```python
from build123d import *

# Parameters (mm, degrees)
SKETCH1_W                      = 80
SKETCH1_H                      = 40
BOSS_EXTRUDE1_DEPTH            = 1000
BOSS_EXTRUDE1_2_DEPTH          = 1000
BOSS_EXTRUDE1_3_DEPTH          = 1000
BOSS_EXTRUDE1_4_DEPTH          = 1000
BOSS_EXTRUDE1_5_DEPTH          = 1000
BOSS_EXTRUDE1_6_DEPTH          = 1000
SKETCH3_W                      = 880
SKETCH3_H                      = 720
SKETCH3_H_2                    = 400
BOSS_EXTRUDE2_DEPTH            = 40
SKETCH4_W                      = 1040
SKETCH4_H                      = 800
SKETCH4_W_2                    = 880
SKETCH4_H_2                    = 720
BOSS_EXTRUDE4_DEPTH            = 40
SKETCH6_W                      = 2000
SKETCH6_H                      = 800
SKETCH6_W_2                    = 880
SKETCH6_H_2                    = 720
BOSS_EXTRUDE5_DEPTH            = 40
SKETCH7_W                      = 80
SKETCH7_H                      = 40
SKETCH8_W                      = 40
SKETCH8_H                      = 40
SKETCH9_W                      = 80
SKETCH9_H                      = 60
BOSS_EXTRUDE6_DEPTH            = 10
F_10_0_10_DIAMETER_HOLE1_D     = 10
F_10_0_10_DIAMETER_HOLE1_DEPTH = 10
MIRROR5_COPY_1_SKETCH_W        = 80
MIRROR5_COPY_1_SKETCH_H        = 60
MIRROR5_COPY_1_DEPTH           = 10
MIRROR5_COPY_2_D               = 10
MIRROR5_COPY_2_DEPTH           = 10


with BuildPart() as part:
    # Sketch1 → Boss-Extrude1 (new body)
    with BuildSketch(Plane(origin=(0, 0, 0), x_dir=(1, 0, 0), z_dir=(0, 1, 0))):
        with Locations((-960, -380)):
            Rectangle(SKETCH1_W, SKETCH1_H)
    extrude(amount=BOSS_EXTRUDE1_DEPTH)



with BuildPart() as body_2:
    # Sketch1 → Boss-Extrude1 2 (new body)
    with BuildSketch(Plane(origin=(0, 0, 0), x_dir=(1, 0, 0), z_dir=(0, 1, 0))):
        with Locations((0, -380)):
            Rectangle(SKETCH1_W, SKETCH1_H)
    extrude(amount=BOSS_EXTRUDE1_2_DEPTH)


with BuildPart() as body_3:
    # Sketch1 → Boss-Extrude1 3 (new body)
    with BuildSketch(Plane(origin=(0, 0, 0), x_dir=(1, 0, 0), z_dir=(0, 1, 0))):
        with Locations((0, 380)):
            Rectangle(SKETCH1_W, SKETCH1_H)
    extrude(amount=BOSS_EXTRUDE1_3_DEPTH)


with BuildPart() as body_4:
    # Sketch1 → Boss-Extrude1 4 (new body)
    with BuildSketch(Plane(origin=(0, 0, 0), x_dir=(1, 0, 0), z_dir=(0, 1, 0))):
        with Locations((-960, 380)):
            Rectangle(SKETCH1_W, SKETCH1_H)
    extrude(amount=BOSS_EXTRUDE1_4_DEPTH)


with BuildPart() as body_5:
    # Sketch1 → Boss-Extrude1 5 (new body)
    with BuildSketch(Plane(origin=(0, 0, 0), x_dir=(1, 0, 0), z_dir=(0, 1, 0))):
        with Locations((960, -380)):
            Rectangle(SKETCH1_W, SKETCH1_H)
    extrude(amount=BOSS_EXTRUDE1_5_DEPTH)


with BuildPart() as body_6:
    # Sketch1 → Boss-Extrude1 6 (new body)
    with BuildSketch(Plane(origin=(0, 0, 0), x_dir=(1, 0, 0), z_dir=(0, 1, 0))):
        with Locations((960, 380)):
            Rectangle(SKETCH1_W, SKETCH1_H)
    extrude(amount=BOSS_EXTRUDE1_6_DEPTH)


with BuildPart() as part_1:
    add(part.part)

    add(body_2.part)  # Boss-Extrude2 merges body 2

    add(body_3.part)  # Boss-Extrude2 merges body 3

    add(body_4.part)  # Boss-Extrude2 merges body 4

    add(body_5.part)  # Boss-Extrude2 merges body 5

    add(body_6.part)  # Boss-Extrude2 merges body 6
    # Sketch3 → Boss-Extrude2 (add)
    with BuildSketch(Plane(origin=(0, 200, 0), x_dir=(-1, 0, 0), z_dir=(0, -1, 0))):
        Polygon((920, -240), (40, -240), (40, -400), (-1000, -400), (-1000, 400), (40, 400), (40, 240), (920, 240), (920, 400), (1000, 400), (1000, -400.075117412), (920, -400.075117412), align=None)
        with Locations((-480, 0)):
            Rectangle(SKETCH3_W, SKETCH3_H, mode=Mode.SUBTRACT)
        with Locations((480, 0)):
            Rectangle(SKETCH3_W, SKETCH3_H_2, mode=Mode.SUBTRACT)
    extrude(amount=BOSS_EXTRUDE2_DEPTH)

    # Sketch4 → Boss-Extrude4 (add)
    with BuildSketch(Plane(origin=(0, 600, 0), x_dir=(-1, 0, 0), z_dir=(0, -1, 0))):
        with Locations((-480, 0)):
            Rectangle(SKETCH4_W, SKETCH4_H)
        with Locations((-480, 0)):
            Rectangle(SKETCH4_W_2, SKETCH4_H_2, mode=Mode.SUBTRACT)
    extrude(amount=BOSS_EXTRUDE4_DEPTH)

    # Sketch6 → Boss-Extrude5 (add)
    with BuildSketch(Plane(origin=(0, 1000, 0), x_dir=(1, 0, 0), z_dir=(0, 1, 0))):
        Rectangle(SKETCH6_W, SKETCH6_H)
        with Locations((-480, 0)):
            Rectangle(SKETCH6_W_2, SKETCH6_H_2, mode=Mode.SUBTRACT)
        with Locations((480, 0)):
            Rectangle(SKETCH6_W_2, SKETCH6_H_2, mode=Mode.SUBTRACT)
    extrude(amount=BOSS_EXTRUDE5_DEPTH)

    # Sweep1: sweep along a curve in space
    with BuildLine() as sweep1_path:
        Line((-960, 200, 360), (-960, 1000, -360))
    # Sketch7 → Sweep1 (sweep)
    with BuildSketch(Plane(origin=(-960, 200, 360), x_dir=(1, 0, 0), z_dir=(0, 0.7432941462471683, -0.6689647316224475))):
        Rectangle(SKETCH7_W, SKETCH7_H)
    sweep(path=sweep1_path.line)

    # Sweep2: sweep along a curve in space
    with BuildLine() as sweep2_path:
        Line((-40, 200, -380), (-920, 1000, -380))
    # Sketch8 → Sweep2 (sweep)
    with BuildSketch(Plane(origin=(-40, 200, -380), x_dir=(0, 0, 1), z_dir=(-0.7399400733959437, 0.6726727939963126, -3.6407320166765e-15))):
        Rectangle(SKETCH8_W, SKETCH8_H)
    sweep(path=sweep2_path.line)

    # Sketch9 → Boss-Extrude6 (add)
    with BuildSketch(Plane.XZ):
        with Locations((960, -330)):
            Rectangle(SKETCH9_W, SKETCH9_H)
    boss_extrude6 = extrude(amount=-BOSS_EXTRUDE6_DEPTH)

    # Ø10.0 (10) Diameter Hole1
    with Locations(Plane(origin=(0, 10, 0), x_dir=(1, 0, 0), z_dir=(0, 1, 0))):
        with Locations((960, 330)):
            f_10_0_10_diameter_hole1 = Hole(F_10_0_10_DIAMETER_HOLE1_D / 2, depth=F_10_0_10_DIAMETER_HOLE1_DEPTH)

    # Mirror4: Boss-Extrude6, Ø10.0 (10) Diameter Hole1 across plane
    add(boss_extrude6.mirror(Plane.XY))
    add(f_10_0_10_diameter_hole1.mirror(Plane.XY), mode=Mode.SUBTRACT)

    # Mirror5: Boss-Extrude6, Ø10.0 (10) Diameter Hole1 across plane
    add(boss_extrude6.mirror(Plane(origin=(0, 0, 0), x_dir=(0, 0, 1), z_dir=(1, 0, 0))))
    add(f_10_0_10_diameter_hole1.mirror(Plane(origin=(0, 0, 0), x_dir=(0, 0, 1), z_dir=(1, 0, 0))), mode=Mode.SUBTRACT)

    # Mirror5 copy 1 sketch → Mirror5 copy 1 (add)
    with BuildSketch(Plane(origin=(0, 0, 0), x_dir=(-1, 0, 0), z_dir=(0, -1, 0))):
        with Locations((960, -330)):
            Rectangle(MIRROR5_COPY_1_SKETCH_W, MIRROR5_COPY_1_SKETCH_H)
    extrude(amount=-MIRROR5_COPY_1_DEPTH)

    # Mirror5 copy 2
    with Locations(Plane(origin=(0, 10, 0), x_dir=(-1, 0, 0), z_dir=(0, 1, 0))):
        with Locations((960, 330)):
            Hole(MIRROR5_COPY_2_D / 2, depth=MIRROR5_COPY_2_DEPTH)


solid = part_1.part
```
Read the model definition and answer for the solid it produces. Units are mm, in the model's axes. A direction names the side the tool comes from. Give positions to 0.01 mm unless a question says otherwise; leave off trailing zeros. Order: outer loops, then holes, each group sorted by start corner. A loop starts at its lowest first (then second) coordinate and runs counter-clockwise, first axis right, second up. Notation, with made-up numbers: (82.5, 43) -> (139.5, 43) arc R13 cw to (139.5, 53) -> close; hole circle Ø4 at (86, 43.5). An arc over 180 degrees is marked (long way). Write item = value, one per line.
1. For faces 1 (the face through (920, 580, 5)), 2 (the face through (40, 377, 380)), 3 (the face through (920, 79, -373)), 4 (the face through (-961, 1000, 9)), determine the directions among +Z, -Z, +X, -X, +Y, -Y from which every point of the face is accessible in a straight line to the end or side of a thin tool.
Numbers:
face_1 = +Y, -Y
face_2 = +Z, -Z
face_3 = +Z, -Z, -Y
face_4 = +X, -X
2. A cutting plane is placed at B-B, the plane y = 798. Count the separate pieces of the cut face and the enclosed holes in it, and give its area (3 significant figures).
Numbers:
separate_pieces = 8
enclosed_holes = 0
area = 25,900 mm²
3. The mould has two halves that part along Z. Classify faces 5 (the face through (40, 797, -380)), 6 (the face through (-1, 79, -360)): +Z half, -Z half, draft (parallel to the pull), parting line (faces both ways), or undercut.
Numbers:
face_5 = draft
face_6 = undercut
4. Straight lines are drawn through the part: line 1 along X through (y, z) = (4.25, 330); line 2 along Z through (x, y) = (960, 3); line 3 along Z through (x, y) = (695, 162). For each, find the intervals that lie inside material, in ascending order.
Numbers:
line_1 = -1000 to -965, -955 to -920, 920 to 955, 965 to 1000
line_2 = -400 to -335, -325 to -300, 300 to 325, 335 to 400
line_3 = -400 to -360, 360 to 400
5. Given pin 1 (20 mm diameter, centred on x = -582, y = 182.5, fed in from -Z), flat-ended and moving along its own axis, determine where the tip first touches the part or whether it passes through.
Numbers:
pin_1 = -240
6. A cutting plane is placed at A-A, the plane x = 346. Write down the section's boundary in (y, z).
Numbers:
outline = (160, -400) -> (200, -400) -> (200, -360) -> (160, -360) -> close; (160, 360) -> (200, 360) -> (200, 400) -> (160, 400) -> close; (560, -400) -> (600, -400) -> (600, -360) -> (560, -360) -> close; (560, 360) -> (600, 360) -> (600, 400) -> (560, 400) -> close; (1000, -400) -> (1040, -400) -> (1040, -360) -> (1000, -360) -> close; (1000, 360) -> (1040, 360) -> (1040, 400) -> (1000, 400) -> close
7. A cutting plane is placed at C-C, the plane x = -515.5. Write down the section's boundary in (y, z), and give its area (3 significant figures).
Numbers:
outline = (160, -240) -> (200, -240) -> (200, -200) -> (160, -200) -> close; (160, 200) -> (200, 200) -> (200, 240) -> (160, 240) -> close; (605.24, -400) -> (659.3, -400) -> (659.3, -360) -> (605.24, -360) -> close; (1000, -400) -> (1040, -400) -> (1040, -360) -> (1000, -360) -> close; (1000, 360) -> (1040, 360) -> (1040, 400) -> (1000, 400) -> close
area = 8,560 mm²
